The model under review builds one solid part; all positions refer to its coordinate system, in mm. A direction names the side the tool comes from. Round coordinates to 2 decimals unless told otherwise and drop trailing zeros. Order: outer loops, then holes, each group sorted by start corner. A loop starts at its lowest first (then second) coordinate and runs counter-clockwise, first axis right, second up.
```python
from build123d import *

# Parameters (mm, degrees)
F1_DEPTH       = 8
F3_DEPTH       = 2.3
F5_D           = 3
F5_CSINK_D     = 5.55
F5_CSINK_ANGLE = 90
F6_R           = 2


with BuildPart() as f1:
    # F0 (on Top) → F1 (new body)
    with BuildSketch(Plane.XY):
        with BuildLine():
            ThreePointArc((-4.141256, 0.7), (4.2, 0), (-4.141256, -0.7))
            Line((-4.141256, -0.7), (-7.467262, -0.7))
            Line((-7.467262, -0.7), (-15.144289, -0.7))
            Line((-15.144289, -0.7), (-15.144289, -4))
            Line((-15.144289, -4), (-6.344289, -4))
            ThreePointArc((-6.344289, -4), (7.5, 0), (-6.344289, 4))
            Line((-6.344289, 4), (-15.144289, 4))
            Line((-15.144289, 4), (-15.144289, 0.7))
            Line((-15.144289, 0.7), (-7.467262, 0.7))
            Line((-7.467262, 0.7), (-4.141256, 0.7))
        make_face()
    extrude(amount=F1_DEPTH)

    # F2 (on face) → F3 (cut)
    with BuildSketch(Plane.XZ.offset(4)):
        Polygon((-12.36087, 1.2), (-9.127708, 1.2), (-7.511127, 4), (-9.127708, 6.8), (-12.36087, 6.8), (-13.97745, 4), align=None)
    extrude(amount=-F3_DEPTH, mode=Mode.SUBTRACT)

    # F5 (through all)
    with Locations(Plane(origin=(0, 4, 0), x_dir=(-1, 0, 0), z_dir=(0, 1, 0))):
        with Locations((10.744289, 4)):
            CounterSinkHole(F5_D / 2, F5_CSINK_D / 2, counter_sink_angle=F5_CSINK_ANGLE)

    # F6
    f6_edges = [f1.edges().sort_by_distance(p)[0] for p in [
        (-4.141256, -0.7, 4),
        (-4.141256, 0.7, 4),
        (-6.344289, -4, 4),
        (-6.344289, 4, 4),
    ]]
    fillet(f6_edges, radius=F6_R)


solid = f1.part
```
(1) Insertion check: pin 1 (3 mm diameter, centred on x = -9.5, z = 4, fed in from -Y); pin 2 (4 mm diameter, centred on x = -10.74, z = 4, fed in from +Y); pin 3 (3 mm diameter, centred on x = -2, z = 2.5, fed in from +Y). Each pin has a flat end and moves straight along its axis. Give the tip position at first contact, or say it passes through.
Data:
pin 1: stops at y = -1.7
pin 2: stops at y = 3.23
pin 3: stops at y = 7.48
(2) Consider section A-A (x = 0). Write out the cut boundary in (y, z).
Data:
outline: (-7.5, 0) - (-4.2, 0) - (-4.2, 8) - (-7.5, 8) - close; (4.2, 0) - (7.5, 0) - (7.5, 8) - (4.2, 8) - close
(3) Consider section B-B (y = 0). Write out the cut boundary in (x, z), and give its area (3 significant figures).
Data:
outline: (4.2, 0) - (7.5, 0) - (7.5, 8) - (4.2, 8) - close
area: 26.4 mm2
(4) Consider section D-D (x = 4.5). Write out the cut boundary in (y, z).
Data:
outline: (-6, 0) - (6, 0) - (6, 8) - (-6, 8) - close
(5) Consider section C-C (z = 4.25). State how many separate pieces and enclosed holes the cut face has, and give its area (3 significant figures).
Data:
separate pieces: 3
enclosed holes: 0
area: 141 mm2
(6) To check wall thickness, follow probe 1 along Y at (x, z) = (0, 3.5); probe 2 along Y at (x, z) = (-13.5, 1); probe 3 along X at (y, z) = (-3, 3.5). State the ranges of each line that lie inside material, in increasing order.
Data:
probe 1: y = -7.5 to -4.2, 4.2 to 7.5
probe 2: y = -4 to -0.7, 0.7 to 4
probe 3: x = -15.14 to -13.69, -7.8 to -2.94, 2.94 to 6.87
(7) Draft analysis for pull direction Y (two halves, no side actions). For faces 5 (the flat face through (-9, -1.7, 5)), 6 (the flat face through (-8.33, -2.87, 2.58)), 7 (the cylindrical face through (4.197, 0.158, 3.944)), state which applies: pulls with the +Y half, pulls with the -Y half, needs draft (parallel to the pull), parting line crosses it, or undercut.
Data:
face 5: pulls with the -Y half
face 6: needs draft
face 7: undercut
(8) For faces 1 (the flat face through (-11, -3, 6.8)), 2 (the flat face through (-13, -4, 6)), 3 (the flat face through (-9, 0.7, 5)), 4 (the cylindrical face through (-4.51, 1.01, 4.06)), list the 3-axis set-ups (+Z, -Z, +X, -X, +Y, -Y) from which the entire face can be reached by the end or side of a thin tool; tool diameter is ignored.
Data:
face 1: -Y
face 2: +Z, -Z, -X, -Y
face 3: +Z, -Z, -X
face 4: +Z, -Z
